```python
from build123d import *

# Parameters (mm, degrees)
EXTRUDE_1_DEPTH     = 39.5
SKETCH_2_R          = 11
EXTRUDE_2_DEPTH     = 2
SKETCH_3_R          = 2.5
EXTRUDE_3_DEPTH     = 20.5
SKETCH_4_R          = 1.5
CUT_EXTRUDE_1_DEPTH = 5
CUT_EXTRUDE_START   = -18
CUT_EXTRUDE_2_DEPTH = 18
SKETCH_6_R          = 4.5
CUT_EXTRUDE_3_DEPTH = 3
CUT_EXTRUDE_START_2 = -3
SKETCH_7_R          = 4.5
SKETCH_7_R_2        = 2.5
CUT_EXTRUDE_4_DEPTH = 3
SKETCH_8_W          = 61.801157568
SKETCH_8_H          = 60.217907666
CUT_EXTRUDE_5_DEPTH = 22


with BuildPart() as part:
    # 草图1 → 凸台-拉伸1 (new body)
    with BuildSketch(Plane.XY):
        Polygon((-17.183766184, 21), (17.183766184, 21), (21, 17.183766184), (21, -17.183766184), (17.183766184, -21), (-17.183766184, -21), (-21, -17.183766184), (-21, 17.183766184), align=None)
    extrude(amount=EXTRUDE_1_DEPTH)

    # 草图2 → 凸台-拉伸2 (add)
    with BuildSketch(Plane(origin=(0, 0, 0), x_dir=(-1, 0, 0), z_dir=(0, 0, -1))):
        Circle(SKETCH_2_R)
    extrude(amount=EXTRUDE_2_DEPTH)

    # 草图3 → 凸台-拉伸3 (add)
    with BuildSketch(Plane(origin=(0, 0, -2), x_dir=(-1, 0, 0), z_dir=(0, 0, -1))):
        Circle(SKETCH_3_R)
    extrude(amount=EXTRUDE_3_DEPTH)

    # 草图4 → 切除-拉伸1 (cut)
    with BuildSketch(Plane(origin=(0, 0, 0), x_dir=(-1, 0, 0), z_dir=(0, 0, -1))):
        with Locations((-15.5, -15.5)):
            Circle(SKETCH_4_R)
        with Locations((-15.5, 15.5)):
            Circle(SKETCH_4_R)
        with Locations((15.5, 15.5)):
            Circle(SKETCH_4_R)
        with Locations((15.5, -15.5)):
            Circle(SKETCH_4_R)
    extrude(amount=-CUT_EXTRUDE_1_DEPTH, mode=Mode.SUBTRACT)

    # 草图5 → 切除-拉伸2 (cut)
    with BuildSketch(Plane(origin=(0, 0, -22.5), x_dir=(-1, 0, 0), z_dir=(0, 0, -1)).offset(CUT_EXTRUDE_START)):
        with BuildLine():
            Line((1.5, 2), (-1.5, 2))
            ThreePointArc((-1.5, 2), (0, 2.5), (1.5, 2))
        make_face()
    extrude(amount=CUT_EXTRUDE_2_DEPTH, mode=Mode.SUBTRACT)

    # 草图6 → 切除-拉伸3 (cut)
    with BuildSketch(Plane.XY.offset(39.5)):
        Circle(SKETCH_6_R)
    extrude(amount=-CUT_EXTRUDE_3_DEPTH, mode=Mode.SUBTRACT)

    # 草图7 → 切除-拉伸4 (cut)
    with BuildSketch(Plane(origin=(0, 0, -2), x_dir=(-1, 0, 0), z_dir=(0, 0, -1)).offset(CUT_EXTRUDE_START_2)):
        with Locations(Location((0, 0, 0), (0, 0, 180))):
            Circle(SKETCH_7_R)
        with Locations(Location((0, 0, 0), (0, 0, 126.869897646))):
            Circle(SKETCH_7_R_2, mode=Mode.SUBTRACT)
    extrude(amount=CUT_EXTRUDE_4_DEPTH, mode=Mode.SUBTRACT)

    # 草图8 → 切除-拉伸5 (cut)
    with BuildSketch(Plane.XY.offset(29.5)):
        Rectangle(SKETCH_8_W, SKETCH_8_H)
        Polygon((21, -14.355339059), (21, 14.355339059), (14.355339059, 21), (-14.355339059, 21), (-21, 14.355339059), (-21, -14.355339059), (-14.355339059, -21), (14.355339059, -21), align=None, mode=Mode.SUBTRACT)
    extrude(amount=-CUT_EXTRUDE_5_DEPTH, mode=Mode.SUBTRACT)


solid = part.part
```
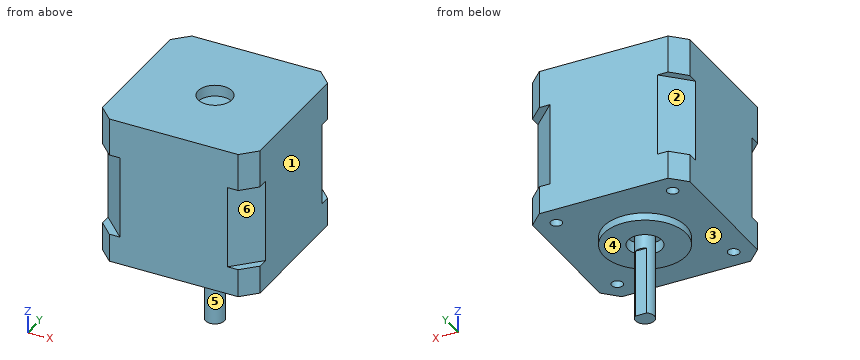
For this review, take the finished solid that the model builds, in its own axes (mm). Face numbers are marked on the shaded views. A direction names the side the tool comes from. Coordinates: 2 decimals unless noted, no trailing zeros. Order: outer loops, then holes, each group sorted by start corner. A loop starts at its lowest first (then second) coordinate and runs counter-clockwise, first axis right, second up. Notation, with made-up numbers: (41.25, 87.5) -> (69.25, 87.5) arc R29 ccw to (69.25, 107.5) -> close; hole circle Ø1 at (40, -3.5). An arc over 180 degrees is marked (long way). Use CSV: the item, a comma, the result in double quotes. Start each with the question number.
Item 1: Draft analysis for pull direction Y (two halves, no side actions). For the marked faces 4, 5 and 6, state which applies: pulls with the +Y half, pulls with the -Y half, needs draft (parallel to the pull), parting line crosses it, or undercut.
Item 2: We need section A-A, the plane z = 26. Give the boundary of the cut face in (x, y).
Item 3: Wall thickness on probe 1 along Y at (x, z) = (0, -1.2); probe 2 along Y at (x, z) = (-15.5, 4); probe 3 along X at (y, z) = (-2, -3): over which ranges is each line inside the solid? List them lowest first.
Item 4: Insertion check: pin 1 (10 mm diameter, centred on y = -5.5, z = -6.5, fed in from +X); pin 2 (0.9 mm diameter, centred on x = 15.5, y = 15.5, fed in from -Z); pin 3 (7.5 mm diameter, centred on x = 18.5, y = -17, fed in from -Z). Each pin has a flat end and moves straight along its axis. Give the tip position at first contact, or say it passes through.
Item 5: We need section B-B, the plane x = 15.5. Give the boundary of the cut face in (y, z), then the cut area to 3 significant figures.
Item 6: We need section D-D, the plane z = 32.5. Give the boundary of the cut face in (x, y).
Item 7: For the marked faces 1, 2 and 3, list the 3-axis set-ups (+Z, -Z, +X, -X, +Y, -Y) from which the entire face can be reached by the end or side of a thin tool; tool diameter is ignored.
Derived:
1,face 4,"needs draft"
1,face 5,"undercut"
1,face 6,"pulls with the -Y half"
2,outline,"(-21, -14.36) -> (-14.36, -21) -> (14.36, -21) -> (21, -14.36) -> (21, 14.36) -> (14.36, 21) -> (-14.36, 21) -> (-21, 14.36) -> close"
3,probe 1,"y = -11 to -4.5, -2.5 to 2.5, 4.5 to 11"
3,probe 2,"y = -21 to -17, -14 to 14, 17 to 21"
3,probe 3,"x = -1.5 to 1.5"
4,pin 1,"stops at x = 10.49"
4,pin 2,"stops at z = 5"
4,pin 3,"stops at z = 0"
5,outline,"(-21, 0) -> (-17, 0) -> (-17, 5) -> (-14, 5) -> (-14, 0) -> (14, 0) -> (14, 5) -> (17, 5) -> (17, 0) -> (21, 0) -> (21, 7.5) -> (19.86, 7.5) -> (19.86, 29.5) -> (21, 29.5) -> (21, 39.5) -> (-21, 39.5) -> (-21, 29.5) -> (-19.86, 29.5) -> (-19.86, 7.5) -> (-21, 7.5) -> close"
5,area,"1,580 mm^2"
6,outline,"(-21, -17.18) -> (-17.18, -21) -> (17.18, -21) -> (21, -17.18) -> (21, 17.18) -> (17.18, 21) -> (-17.18, 21) -> (-21, 17.18) -> close"
7,face 1,"+Z, -Z, +X, +Y, -Y"
7,face 2,"-X, +Y"
7,face 3,"-Z"
